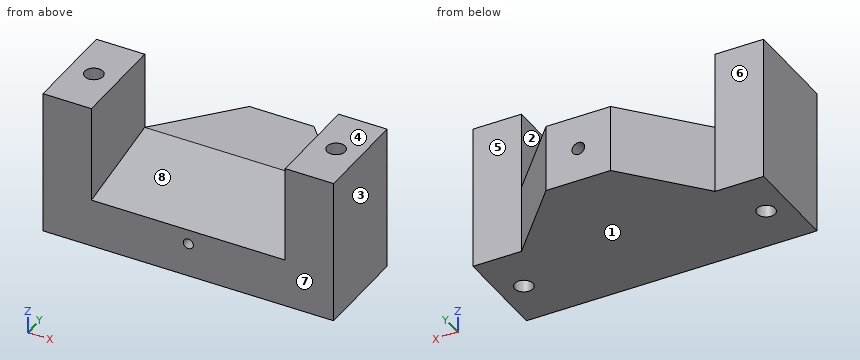
Autodesk Inventor part; units mm, degrees
ref_plane "YZ Plane" through (0, 0, 0) normal (1, 0, 0) x (0, 1, 0)
ref_plane "XZ Plane" through (0, 0, 0) normal (0, 1, 0) x (-1, 0, 0)
ref_plane "XY Plane" through (0, 0, 0) normal (0, 0, 1) x (1, 0, 0)
sketch "Sketch1" plane through (0, 0, 0) normal (0, 1, 0) x (-1, 0, 0)
  line L0 (0, 0) -> (12.7, 0)
  line L1 (12.7, 0) -> (12.7, 38.1)
  line L2 (12.7, 38.1) -> (0, 38.1)
  line L3 (0, 38.1) -> (0, 0)
  line L4 (12.7, 0) -> (63.5, 0)
  line L5 (63.5, 0) -> (63.5, 12.7)
  line L6 (63.5, 12.7) -> (12.7, 12.7)
  line L7 (12.7, 12.7) -> (12.7, 0)
  line L8 (63.5, 0) -> (76.2, 0)
  line L9 (76.2, 0) -> (76.2, 38.1)
  line L10 (76.2, 38.1) -> (63.5, 38.1)
  line L11 (63.5, 38.1) -> (63.5, 0)
  dimension "d0" = 38.1
  dimension "d1" = 38.1
  dimension "d2" = 12.7
  dimension "d3" = 12.7
  dimension "d5" = 50.8
  dimension "d6" = 12.7
extrude "Extrusion1" add sketch "Sketch1" along normal blind 25.4
sketch "Sketch2" plane through (-63.5, 0, 38.1) normal (1, 0, 0) x (0, 0, -1)
  line L0 (25.4, 0) -> (25.4, 25.4)
  line L1 (25.4, 0) -> (20.32, 25.4)
  line L2 (0, 25.4) -> (25.4, 25.4)
  point P0 (38.1, 0)
  dimension "d9" = 5.08
extrude "Extrusion2" add sketch "Sketch2" along normal blind 50.8
sketch "Sketch3" plane through (-76.2, 0, 38.1) normal (0, 0, 1) x (1, 0, 0)
  line L0 (0, 25.4) -> (12.7, 25.4)
  line L1 (0, 0) -> (0, 25.4)
  line L2 (63.5, 25.4) -> (76.2, 25.4)
  line L3 (76.2, 0) -> (76.2, 25.4)
  point P0 (6.35, 12.7)
  point P1 (69.85, 12.7)
  dimension "d12" = 12.7
  dimension "d13" = 25.4
  dimension "d14" = 6.35
  dimension "d15" = 12.7
  dimension "d16" = 12.7
  dimension "d17" = 25.4
  dimension "d18" = 12.7
  dimension "d19" = 6.35
hole "Hole1" at (-69.85, 12.7, 38.1) at (-6.35, 12.7, 38.1) direction (0, 0, -1) diameter 4.7625 end through all
sketch "Sketch4" plane through (0, 25.4, 0) normal (0, 1, 0) x (1, 0, 0)
  line L0 (0, 0) -> (-76.2, 0)
  line L1 (0, -38.1) -> (0, 0)
  line L2 (-12.7, -17.78) -> (-12.7, -38.1)
  point P0 (-38.1, -8.89)
  dimension "d27" = 38.1
  dimension "d28" = 20.32
  dimension "d29" = 76.2
  dimension "d30" = 38.1
  dimension "d31" = 8.89
hole "Hole2" at (-38.1, 25.4, 8.89) direction (0, -1, 0) diameter 2.6416 end through all
sketch "Sketch5" plane through (0, 25.4, 0) normal (0, 1, 0) x (1, 0, 0)
  line L0 (-63.5, -17.78) -> (-12.7, -17.78)
  line L1 (0, 0) -> (-76.2, 0)
  line L2 (-63.5, -17.78) -> (-12.7, -17.78)
  line L3 (-12.7, -17.78) -> (-12.7, 0)
  line L4 (-12.7, 0) -> (-63.5, 0)
  line L5 (-63.5, 0) -> (-63.5, -17.78)
  line L6 (-12.7, -38.1) -> (0, -38.1)
  line L7 (0, -38.1) -> (0, 0)
  dimension "d39" = 12.7
  dimension "d40" = 12.7
extrude "Extrusion3" add sketch "Sketch5" along normal blind 19.05
sketch "Sketch6" plane through (-63.5, 25.4, 17.78) normal (0, 0, 1) x (1, 0, 0)
  line L0 (0, 0) -> (50.8, 0)
  line L1 (0, 0) -> (16.9333, 19.05)
  line L2 (50.8, 19.05) -> (0, 19.05)
  line L3 (63.5, 0) -> (50.8, 0)
  line L4 (50.8, 0) -> (33.8667, 19.05)
  line L5 (0, 0) -> (0, 19.05)
  line L6 (0, 0) -> (50.8, 0)
  line L7 (50.8, 0) -> (50.8, 19.05)
  line L8 (0, 19.05) -> (50.8, 19.05)
  line L9 (0, 0) -> (0, 19.05)
  point P0 (63.5, -25.4)
  dimension "d43" = 50.8
  dimension "d44" = 16.9333
  dimension "d45" = 16.9333
extrude "Extrusion4" cut sketch "Sketch6" against normal blind 19.05 contours L5 L2 L1 | L4 L2 L7
sketch "Sketch7" plane through (0, 44.45, 0) normal (0, 1, 0) x (1, 0, 0)
  circle A0 centre (-38.1, -8.89) radius 1.3208
  point P0 (0, 0)
hole "Hole3" at (-38.1, 44.45, 8.89) direction (0, -1, 0) diameter 3.302 depth 12.2936 tip angle 118
equation "\"d1\" = d0"
equation "\"d3\" = d2"
equation "\"d40\" = d39"
equation "\"d44\" = 0.333333 * d43"
equation "\"d45\" = 0.333333 * d43"
properties part number "sliding piece for grabber"
Check sheet for the modelled part. Datum: model origin and axes. Units: mm. Face numbers are marked on the shaded views. A direction names the side the tool comes from. Give positions to 0.01 mm unless a question says otherwise; leave off trailing zeros. Write each loop counter-clockwise with the first axis right and the second up, starting at its lowest first coordinate (ties: lowest second). Pieces come first, ordered by that corner, then holes. Notation, with made-up numbers: (-30, 48) -> (-1, 48) arc R21 ccw to (-1, 86) -> close; hole circle Ø11 at (-39.75, 53.25). An arc over 180 degrees is marked (long way). Write item = value, one per line.
Item 1: Sectioned sample at B-B on y = 12.7. Record the boundary of the cut face in (x, z).
Output:
outline = (-76.2, 0) -> (-72.23, 0) -> (-72.23, 38.1) -> (-76.2, 38.1) -> close; (-67.47, 0) -> (-8.73, 0) -> (-8.73, 38.1) -> (-12.7, 38.1) -> (-12.7, 15.24) -> (-63.5, 15.24) -> (-63.5, 38.1) -> (-67.47, 38.1) -> close; (-3.97, 0) -> (0, 0) -> (0, 38.1) -> (-3.97, 38.1) -> close; hole circle Ø2.64 at (-38.1, 8.89)
Item 2: Gauge pin test, flat ends, axial feed: pin 1 (8 mm diameter, centred on y = 33, z = 14, fed in from -X); pin 2 (4 mm diameter, centred on x = -15.5, z = 28, fed in from +Y); pin 3 (9.5 mm diameter, centred on x = -46, y = 32.5, fed in from +Z); pin 4 (10 mm diameter, centred on x = -7, z = 18.5, fed in from +Y). Record the tip position at first contact, or that the pin passes through.
Output:
pin_1 = -60.3
pin_2 = through
pin_3 = 17.78
pin_4 = 25.4
Item 3: Sectioned sample at A-A on z = 21. Record the boundary of the cut face in (x, y), and give its area (3 significant figures).
Output:
outline = (-76.2, 0) -> (-63.5, 0) -> (-63.5, 25.4) -> (-76.2, 25.4) -> close; (-12.7, 0) -> (0, 0) -> (0, 25.4) -> (-12.7, 25.4) -> close; hole circle Ø4.76 at (-69.85, 12.7); hole circle Ø4.76 at (-6.35, 12.7)
area = 610 mm^2
Item 4: Scan lines: probe 1 along X at (y, z) = (12.7, 20); probe 2 along X at (y, z) = (12.7, 13); probe 3 along Z at (x, y) = (-38.1, 38.5). Record each from-to range of solid material in increasing order. Write a range as from..to.
Output:
probe_1 = -76.2..-72.23, -67.47..-63.5, -12.7..-8.73, -3.97..0
probe_2 = -76.2..-72.23, -67.47..-8.73, -3.97..0
probe_3 = 0..7.24, 10.54..17.78
Item 5: Tool access check on the marked faces 4, 5, 6, 7 and 8. Record the directions out of +Z, -Z, +X, -X, +Y, -Y that give a thin tool (end or side, any length) a straight path to the whole face; none if there is none.
Output:
face_4 = +Z, +X, -X, +Y, -Y
face_5 = +Z, -Z, +X, +Y
face_6 = +Z, -Z, -X, +Y
face_7 = +Z, -Z, +X, -X, -Y
face_8 = +Z, -Y
Item 6: Release check for a two-part mould opening along X. For the marked faces 1, 2 and 3 record: +X half, -X half, draft (parallel to the pull), parting line (faces both ways), or undercut.
Output:
face_1 = draft
face_2 = undercut
face_3 = +X half
Item 7: Sectioned sample at C-C on z = 4.5. Record the boundary of the cut face in (x, y).
Output:
outline = (-76.2, 0) -> (0, 0) -> (0, 25.4) -> (-12.7, 25.4) -> (-29.63, 44.45) -> (-46.57, 44.45) -> (-63.5, 25.4) -> (-76.2, 25.4) -> close; hole circle Ø4.76 at (-69.85, 12.7); hole circle Ø4.76 at (-6.35, 12.7)
Item 8: Sectioned sample at D-D on x = -69.85. Record the boundary of the cut face in (y, z).
Output:
outline = (0, 0) -> (10.32, 0) -> (10.32, 38.1) -> (0, 38.1) -> close; (15.08, 0) -> (25.4, 0) -> (25.4, 38.1) -> (15.08, 38.1) -> close
